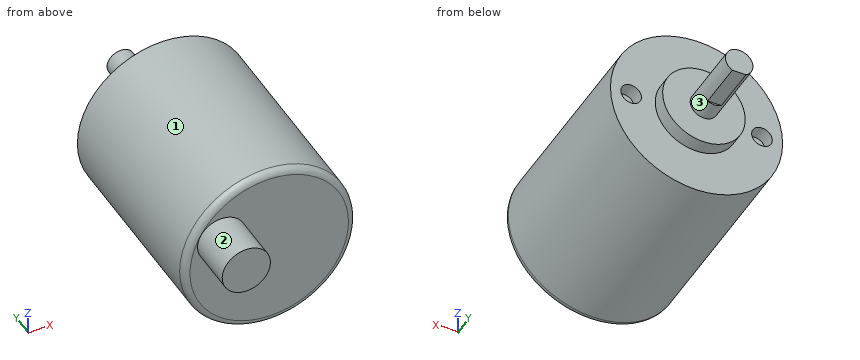
```python
from build123d import *

# Parameters (mm, degrees)
SKETCH_1_R          = 12.5
EXTRUDE_1_DEPTH     = 30
FILLET_1_R          = 1
SKETCH_2_R          = 6
EXTRUDE_2_DEPTH     = 2.1
SKETCH_3_R          = 1.5
CUT_EXTRUDE_1_DEPTH = 2.1
SKETCH_4_R          = 2
EXTRUDE_3_DEPTH     = 10
CUT_EXTRUDE_START   = -7
CUT_EXTRUDE_2_DEPTH = 7
SKETCH_6_R          = 3.5
EXTRUDE_4_DEPTH     = 7


with BuildPart() as part:
    # 草图1 → 凸台-拉伸1 (new body)
    with BuildSketch(Plane(origin=(0, 0, 0), x_dir=(1, 0, 0), z_dir=(0, 1, 0))):
        with Locations(Location((0, 0, 0), (0, 0, 270))):
            Circle(SKETCH_1_R)
    extrude(amount=EXTRUDE_1_DEPTH)

    # 圆角1
    fillet_1_edges = [part.edges().sort_by_distance(p)[0] for p in [
        (0, 0, -12.5),
    ]]
    fillet(fillet_1_edges, radius=FILLET_1_R)

    # 草图2 → 凸台-拉伸2 (add)
    with BuildSketch(Plane(origin=(0, 30, 0), x_dir=(1, 0, 0), z_dir=(0, 1, 0))):
        with Locations(Location((0, 0, 0), (0, 0, 270))):
            Circle(SKETCH_2_R)
    extrude(amount=EXTRUDE_2_DEPTH)

    # 草图3 → 切除-拉伸1 (cut)
    with BuildSketch(Plane(origin=(0, 30, 0), x_dir=(1, 0, 0), z_dir=(0, 1, 0))):
        with Locations(Location((-9.5, 0, 0), (0, 0, 270))):
            Circle(SKETCH_3_R)
        with Locations(Location((9.5, 0, 0), (0, 0, 270))):
            Circle(SKETCH_3_R)
    extrude(amount=-CUT_EXTRUDE_1_DEPTH, mode=Mode.SUBTRACT)

    # 草图4 → 凸台-拉伸3 (add)
    with BuildSketch(Plane(origin=(0, 32.1, 0), x_dir=(1, 0, 0), z_dir=(0, 1, 0))):
        with Locations(Location((0, 0, 0), (0, 0, 270))):
            Circle(SKETCH_4_R)
    extrude(amount=EXTRUDE_3_DEPTH)

    # 草图5 → 切除-拉伸2 (cut)
    with BuildSketch(Plane(origin=(0, 42.1, 0), x_dir=(1, 0, 0), z_dir=(0, 1, 0)).offset(CUT_EXTRUDE_START)):
        with BuildLine():
            Line((-0.99729895, 1.733607454), (0.99729895, 1.733607454))
            ThreePointArc((0.99729895, 1.733607454), (0, 2), (-0.99729895, 1.733607454))
        make_face()
    extrude(amount=CUT_EXTRUDE_2_DEPTH, mode=Mode.SUBTRACT)

    # 草图6 → 凸台-拉伸4 (add)
    with BuildSketch(Plane.XZ):
        with Locations(Location((-6.913670465, 3.996713823, 0), (0, 0, 90))):
            Circle(SKETCH_6_R)
    extrude(amount=EXTRUDE_4_DEPTH)


solid = part.part
```
Model file for the job. Use its own axes, mm. Face numbers are marked on the shaded views. A direction names the side the tool comes from. Give positions to 0.01 mm unless a question says otherwise; leave off trailing zeros. Write each loop counter-clockwise with the first axis right and the second up, starting at its lowest first coordinate (ties: lowest second). Pieces come first, ordered by that corner, then holes. Notation, with made-up numbers: M 27,-18 L 47,-18 A17 ccw 47,-4 Z; hole C 7.25,78.25 d8. An arc over 180 degrees is marked long. Use a Markdown table: item, result.
1) Cut at A-A (z = 0). List the corners of the cut face in (x, y), and give its area (3 significant figures).
Responses:
| item | result |
|---|---|
| outline | M -12.5,1 A1 ccw -11.5,0 L 11.5,0 A1 ccw 12.5,1 L 12.5,30 L 11,30 L 11,27.9 L 8,27.9 L 8,30 L 6,30 L 6,32.1 L 2,32.1 L 2,42.1 L -2,42.1 L -2,32.1 L -6,32.1 L -6,30 L -8,30 L -8,27.9 L -11,27.9 L -11,30 L -12.5,30 Z |
| area | 802 mm2 |
2) Pin check, flat tips, straight feed: pin 1 (1.5 mm diameter, centred on y = 22, z = 3.5, fed in from -X); pin 2 (6 mm diameter, centred on y = 30, z = 8.5, fed in from -X) (3 decimals); pin 3 (3 mm diameter, centred on x = 8.5, z = -3, fed in from -Y). Stop position of each tip, or through.
Responses:
| item | result |
|---|---|
| pin 1 | stops at x = -12.19 |
| pin 2 | stops at x = -11.225 |
| pin 3 | stops at y = 0 |
3) Tool access for the marked faces 1, 2 and 3: list every direction of +Z, -Z, +X, -X, +Y, -Y with a clear straight run to the whole face (end or side of a thin tool).
Responses:
| item | result |
|---|---|
| face 1 | +Y, -Y |
| face 2 | -Y |
| face 3 | +Y |
4) Drill centre lines: line 1 (X direction, y = 28.4, z = 0); line 2 (Y direction, x = 4.5, z = -2.75); line 3 (Y direction, x = -0.5, z = 7.75). Where is each one in solid material? Low to high. Write a range as from..to.
Responses:
| item | result |
|---|---|
| line 1 | x = -12.5..-11, -8..8, 11..12.5 |
| line 2 | y = 0..32.1 |
| line 3 | y = 0..30 |
5) Cut at B-B (y = 25.5). List the corners of the cut face in (x, z).
Responses:
| item | result |
|---|---|
| outline | C 0,0 d25 |
